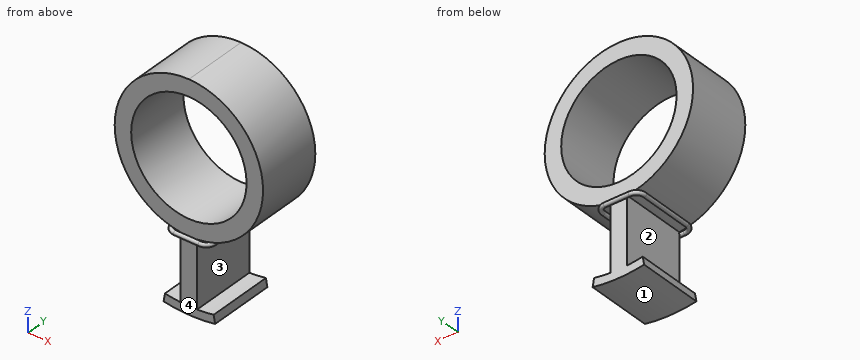
```python
from build123d import *

# Parameters (mm, degrees)
SKETCH1_R           = 90
SKETCH1_R_2         = 70
BOSS_EXTRUDE1_DEPTH = 80
BOSS_EXTRUDE2_DEPTH = 80
SKETCH3_R           = 2.5


with BuildPart() as part:
    # Sketch1 → Boss-Extrude1 (new body)
    with BuildSketch(Plane(origin=(0, 0, 0), x_dir=(1, 0, 0), z_dir=(0, 1, 0))):
        with Locations(Location((0, 0, 0), (0, 0, 270))):
            Circle(SKETCH1_R)
        with Locations(Location((0, 0, 0), (0, 0, 270))):
            Circle(SKETCH1_R_2, mode=Mode.SUBTRACT)
    extrude(amount=BOSS_EXTRUDE1_DEPTH)

    # Sketch1_3 → Boss-Extrude2 (add)
    with BuildSketch(Plane(origin=(0, 0, 0), x_dir=(1, 0, 0), z_dir=(0, 1, 0))):
        with BuildLine():
            ThreePointArc((31.838312344, 177.161852178), (0.590784056, 179.999030481), (-30.674694906, 177.367029327))
            Line((-30.674694906, 177.367029327), (-28.970545189, 167.513305476))
            ThreePointArc((-28.970545189, 167.513305476), (-19.516080985, 168.876056867), (-10, 169.705627485))
            Line((-10, 169.705627485), (-10, 89.4427191))
            ThreePointArc((-10, 89.4427191), (0, 90), (10, 89.4427191))
            Line((10, 89.4427191), (10, 169.705627485))
            ThreePointArc((10, 169.705627485), (20.070249656, 168.811092878), (30.069517214, 167.319527057))
            Line((30.069517214, 167.319527057), (31.838312344, 177.161852178))
        make_face()
    extrude(amount=BOSS_EXTRUDE2_DEPTH)

    # Sweep1: sweep along a path in Sketch2
    with BuildLine(Plane.XY.offset(-91)) as sweep1_path:
        Line((15, -2.25), (-15, -2.25))
        ThreePointArc((-15, -2.25), (-22.071067812, 0.678932188), (-25, 7.75))
        Line((-25, 7.75), (-25, 72.25))
        ThreePointArc((-25, 72.25), (-22.071067812, 79.321067812), (-15, 82.25))
        Line((-15, 82.25), (15, 82.25))
        ThreePointArc((15, 82.25), (22.071067812, 79.321067812), (25, 72.25))
        Line((25, 72.25), (25, 7.75))
        ThreePointArc((25, 7.75), (22.071067812, 0.678932188), (15, -2.25))
    # Sketch3 → Sweep1 (sweep)
    with BuildSketch(Plane(origin=(0, 0, 0), x_dir=(0, 0, -1), z_dir=(1, 0, 0))):
        with Locations((91, 82.25)):
            Circle(SKETCH3_R)
    sweep(path=sweep1_path.line)


solid = part.part
```
Input: part model. Units: mm. Frame: model coordinates. Face numbers are marked on the shaded views. Round coordinates to 2 decimals unless told otherwise and drop trailing zeros. Loops run counter-clockwise (first coordinate to the right, second up) from the corner with the lowest first, then second, coordinate; pieces in that order, holes last.
1) Section query C-C on z = 0. Return the cut outline in (x, y).
Ans:
outline: (-90, 0) - (-70, 0) - (-70, 80) - (-90, 80) - close; (70, 0) - (90, 0) - (90, 80) - (70, 80) - close
2) Section query A-A on y = 21. Return the cut outline in (x, z), plus the area to 3 significant figures.
Ans:
outline: (-30.67, -177.37) arc R180 ccw to (31.84, -177.16) - (30.07, -167.32) arc R170 cw to (10, -169.71) - (10, -89.44) arc R90 ccw (long way) to (-10, -89.44) - (-10, -169.71) arc R170 cw to (-28.97, -167.51) - close; circle Ø5 at (-25, -91); circle Ø5 at (25, -91); hole circle Ø140 at (0, 0)
area: 12,300 mm2
3) Material intervals for line 1 (X direction, y = 38, z = 0); line 2 (Z direction, x = 16, y = 69.5); line 3 (Z direction, x = 20, y = 27), sorted ascending.
Ans:
line 1: x = -90 to -70, 70 to 90
line 2: z = -179.29 to -169.25, -88.57 to -68.15, 68.15 to 88.57
line 3: z = -178.89 to -168.82, -87.75 to -67.08, 67.08 to 87.75
4) Section query D-D on x = 19. Count the separate pieces of the cut face and the enclosed holes in it, plus the area to 3 significant figures.
Ans:
separate pieces: 5
enclosed holes: 0
area: 4,140 mm2
5) Section query B-B on x = 54. Return the cut outline in (y, z), plus the area to 3 significant figures.
Ans:
outline: (0, -72) - (80, -72) - (80, -44.54) - (0, -44.54) - close; (0, 44.54) - (80, 44.54) - (80, 72) - (0, 72) - close
area: 4,390 mm2
6) Pin query (flat end, axial travel): pin 1 (1 mm diameter, centred on y = 29, z = 26.5, fed in from +X); pin 2 (1.5 mm diameter, centred on y = 50.5, z = 31.5, fed in from -X); pin 3 (1.5 mm diameter, centred on x = 15, y = 50, fed in from +Z). Return the tip coordinate at first contact, or that it passes through.
Ans:
pin 1: stops at x = 86.16
pin 2: stops at x = -84.58
pin 3: stops at z = 88.86
7) Pull-direction query (Z, two-part tool) for the marked faces 1, 2, 3 and 4; classes: released by +Z, released by -Z, zero draft, split by the parting line, or undercut.
Ans:
face 1: released by -Z
face 2: undercut
face 3: undercut
face 4: zero draft
